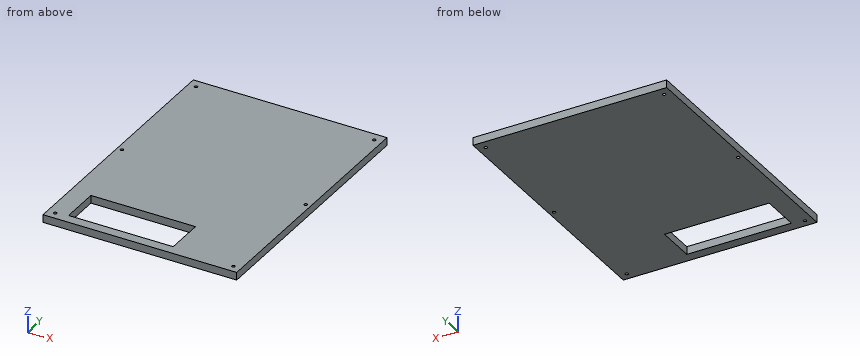
from build123d import *

# Parameters (mm, degrees)
CROQUIS1_W              = 250
CROQUIS1_H              = 336.42
SALIENTE_EXTRUIR1_DEPTH = 10
CORTAR_EXTRUIR1_REACH   = 12
CROQUIS2_R              = 2
CORTAR_EXTRUIR2_REACH   = 12
CROQUIS3_W              = 135
CROQUIS3_H              = 50


with BuildPart() as part:
    # Croquis1 → Saliente-Extruir1 (new body)
    with BuildSketch(Plane.XY):
        Rectangle(CROQUIS1_W, CROQUIS1_H)
    extrude(amount=SALIENTE_EXTRUIR1_DEPTH)

    # Croquis2 → Cortar-Extruir1 (cut, up to next)
    with BuildSketch(Plane(origin=(0, 0, 0), x_dir=(-1, 0, 0), z_dir=(0, 0, -1)), mode=Mode.PRIVATE) as cortar_extruir1_sk1:
        with Locations((115, 156.881750805)):
            Circle(CROQUIS2_R)
    cortar_extruir1_tool1 = extrude(cortar_extruir1_sk1.sketch, amount=-CORTAR_EXTRUIR1_REACH, mode=Mode.PRIVATE) & part.part
    add(cortar_extruir1_tool1.solids().sort_by_distance((-115, 156.881751, 0))[0], mode=Mode.SUBTRACT)
    # Croquis2 → Cortar-Extruir1 (cut, up to next)
    with BuildSketch(Plane(origin=(0, 0, 0), x_dir=(-1, 0, 0), z_dir=(0, 0, -1)), mode=Mode.PRIVATE) as cortar_extruir1_sk2:
        with Locations((-115, 156.881750805)):
            Circle(CROQUIS2_R)
    cortar_extruir1_tool2 = extrude(cortar_extruir1_sk2.sketch, amount=-CORTAR_EXTRUIR1_REACH, mode=Mode.PRIVATE) & part.part
    add(cortar_extruir1_tool2.solids().sort_by_distance((115, 156.881751, 0))[0], mode=Mode.SUBTRACT)
    # Croquis2 → Cortar-Extruir1 (cut, up to next)
    with BuildSketch(Plane(origin=(0, 0, 0), x_dir=(-1, 0, 0), z_dir=(0, 0, -1)), mode=Mode.PRIVATE) as cortar_extruir1_sk3:
        with Locations((-118.75, -2.472724195)):
            Circle(CROQUIS2_R)
    cortar_extruir1_tool3 = extrude(cortar_extruir1_sk3.sketch, amount=-CORTAR_EXTRUIR1_REACH, mode=Mode.PRIVATE) & part.part
    add(cortar_extruir1_tool3.solids().sort_by_distance((118.75, -2.472724, 0))[0], mode=Mode.SUBTRACT)
    # Croquis2 → Cortar-Extruir1 (cut, up to next)
    with BuildSketch(Plane(origin=(0, 0, 0), x_dir=(-1, 0, 0), z_dir=(0, 0, -1)), mode=Mode.PRIVATE) as cortar_extruir1_sk4:
        with Locations((118.75, -2.472724195)):
            Circle(CROQUIS2_R)
    cortar_extruir1_tool4 = extrude(cortar_extruir1_sk4.sketch, amount=-CORTAR_EXTRUIR1_REACH, mode=Mode.PRIVATE) & part.part
    add(cortar_extruir1_tool4.solids().sort_by_distance((-118.75, -2.472724, 0))[0], mode=Mode.SUBTRACT)
    # Croquis2 → Cortar-Extruir1 (cut, up to next)
    with BuildSketch(Plane(origin=(0, 0, 0), x_dir=(-1, 0, 0), z_dir=(0, 0, -1)), mode=Mode.PRIVATE) as cortar_extruir1_sk5:
        with Locations((-115, -158.388099131)):
            Circle(CROQUIS2_R)
    cortar_extruir1_tool5 = extrude(cortar_extruir1_sk5.sketch, amount=-CORTAR_EXTRUIR1_REACH, mode=Mode.PRIVATE) & part.part
    add(cortar_extruir1_tool5.solids().sort_by_distance((115, -158.388099, 0))[0], mode=Mode.SUBTRACT)
    # Croquis2 → Cortar-Extruir1 (cut, up to next)
    with BuildSketch(Plane(origin=(0, 0, 0), x_dir=(-1, 0, 0), z_dir=(0, 0, -1)), mode=Mode.PRIVATE) as cortar_extruir1_sk6:
        with Locations((115, -158.388099131)):
            Circle(CROQUIS2_R)
    cortar_extruir1_tool6 = extrude(cortar_extruir1_sk6.sketch, amount=-CORTAR_EXTRUIR1_REACH, mode=Mode.PRIVATE) & part.part
    add(cortar_extruir1_tool6.solids().sort_by_distance((-115, -158.388099, 0))[0], mode=Mode.SUBTRACT)

    # Croquis3 → Cortar-Extruir2 (cut, up to next)
    with BuildSketch(Plane(origin=(0, 0, 0), x_dir=(-1, 0, 0), z_dir=(0, 0, -1)), mode=Mode.PRIVATE) as cortar_extruir2_sk1:
        with Locations((31.860667122, -130.421960957)):
            Rectangle(CROQUIS3_W, CROQUIS3_H)
    cortar_extruir2_tool1 = extrude(cortar_extruir2_sk1.sketch, amount=-CORTAR_EXTRUIR2_REACH, mode=Mode.PRIVATE) & part.part
    add(cortar_extruir2_tool1.solids().sort_by_distance((-31.860667, -130.421961, 0))[0], mode=Mode.SUBTRACT)


solid = part.part
Design review of the part built by this model. Coordinates are the model's own, in mm. Give positions to 0.01 mm unless a question says otherwise; leave off trailing zeros. Loops run counter-clockwise (first coordinate to the right, second up) from the corner with the lowest first, then second, coordinate; pieces in that order, holes last. Notation, with made-up numbers: M 8.25,12 L 45.25,12 A29 ccw 45.25,49 Z; hole C 77,-28.5 d5. An arc over 180 degrees is marked long. One line per question, with ' | ' between items. Start each with the question number.
1. Add section B-B (x = -83.5). Write out the cut boundary in (y, z), plus the area to 3 significant figures.
2. Insertion check: P1, Ø6.5, axis at x = 118.75, y = -2.47, coming from the -Z side. The pin has a flat end and moves straight along its axis. Give the tip position at first contact, or say it passes through.
3. To check wall thickness, follow L1, parallel to Y at x = 31, z = 5; L2, parallel to Y at x = 115, z = 2.5; L3, parallel to X at y = -111, z = 7.5. State the ranges of each line that lie inside material, in increasing order.
4. Add section C-C (z = 7). Write out the cut boundary in (x, y).
5. Add section A-A (y = -140). Write out the cut boundary in (x, z), plus the area to 3 significant figures.
Worked out:
1) outline: M -168.21,0 L -155.42,0 L -155.42,10 L -168.21,10 Z; M -105.42,0 L 168.21,0 L 168.21,10 L -105.42,10 Z | area: 2,860 mm²
2) P1: stops at z = 0
3) L1: y = -168.21 to -155.42, -105.42 to 168.21 | L2: y = -168.21 to -160.39, -156.39 to 154.88, 158.88 to 168.21 | L3: x = -125 to -99.36, 35.64 to 125
4) outline: M -125,-168.21 L 125,-168.21 L 125,168.21 L -125,168.21 Z; hole C -118.75,-2.47 d4; hole C -115,-158.39 d4; hole C -115,156.88 d4; hole M -99.36,-155.42 L 35.64,-155.42 L 35.64,-105.42 L -99.36,-105.42 Z; hole C 115,-158.39 d4; hole C 115,156.88 d4; hole C 118.75,-2.47 d4
5) outline: M -125,0 L -99.36,0 L -99.36,10 L -125,10 Z; M 35.64,0 L 125,0 L 125,10 L 35.64,10 Z | area: 1,150 mm²
